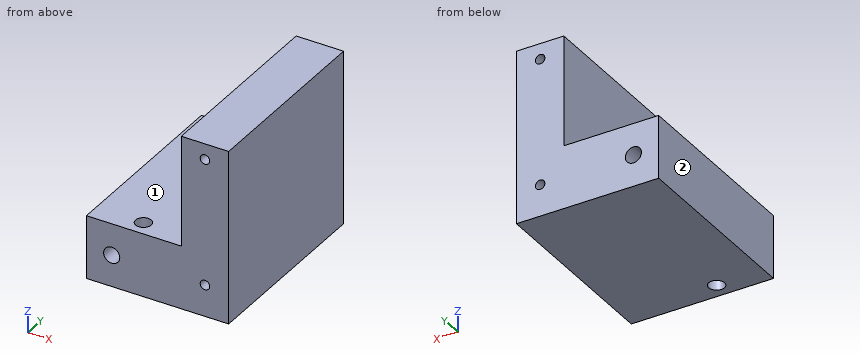
from build123d import *

# Parameters (mm, degrees)
SKETCH1_W           = 15
SKETCH1_H           = 55
SKETCH1_R           = 1.5
SKETCH1_W_2         = 30
SKETCH1_H_2         = 20
SKETCH1_R_2         = 2.55
BOSS_EXTRUDE1_DEPTH = 60
SKETCH2_R           = 2.5
CUT_EXTRUDE1_DEPTH  = 20


with BuildPart() as part:
    # Sketch1 → Boss-Extrude1 (new body)
    # profile 1 of 2: a face of its own
    with BuildSketch(Plane(origin=(0, 0, 0), x_dir=(1, 0, 0), z_dir=(0, 1, 0))):
        Rectangle(SKETCH1_W, SKETCH1_H)
        with Locations(Location((0, -22.5, 0), (0, 0, 270))):
            Circle(SKETCH1_R, mode=Mode.SUBTRACT)
        with Locations(Location((0, 17.5, 0), (0, 0, 270))):
            Circle(SKETCH1_R, mode=Mode.SUBTRACT)
    # profile 2 of 2: a face of its own
    with BuildSketch(Plane(origin=(0, 0, 0), x_dir=(1, 0, 0), z_dir=(0, 1, 0))):
        with Locations((-22.5, 17.5)):
            Rectangle(SKETCH1_W_2, SKETCH1_H_2)
        with Locations(Location((-29.5, 17.5, 0), (0, 0, 270))):
            Circle(SKETCH1_R_2, mode=Mode.SUBTRACT)
    extrude(amount=BOSS_EXTRUDE1_DEPTH)

    # Sketch2 → Cut-Extrude1 (cut)
    with BuildSketch(Plane(origin=(0, 0, -27.5), x_dir=(-1, 0, 0), z_dir=(0, 0, -1))):
        with Locations((22.5, 5)):
            Circle(SKETCH2_R)
    extrude(amount=-CUT_EXTRUDE1_DEPTH, mode=Mode.SUBTRACT)


solid = part.part
Geometry check sheet. Reference: the model listing, model coordinates, mm. Face numbers are marked on the shaded views. A direction names the side the tool comes from. Give positions to 0.01 mm unless a question says otherwise; leave off trailing zeros. Order: outer loops, then holes, each group sorted by start corner. A loop starts at its lowest first (then second) coordinate and runs counter-clockwise, first axis right, second up.
1. Sectioned sample at A-A (y = 5). Record the boundary of the cut face in (x, z).
Completed:
outline: (-37.5, -27.5) - (-25, -27.5) - (-25, -7.5) - (-37.5, -7.5) - close; (-20, -27.5) - (7.5, -27.5) - (7.5, 27.5) - (-7.5, 27.5) - (-7.5, -7.5) - (-20, -7.5) - close; hole circle Ø5.1 at (-29.5, -17.5); hole circle Ø3 at (0, -17.5); hole circle Ø3 at (0, 22.5)
2. Depth check by flat-ended pin: pin 1 (1.8 mm diameter, centred on x = 0, z = -17.5, fed in from -Y); pin 2 (4 mm diameter, centred on x = -30, z = -21, fed in from -Y); pin 3 (4 mm diameter, centred on y = 31.5, z = 13.5, fed in from -X); pin 4 (8 mm diameter, centred on x = -14.5, y = 52, fed in from +Z). Enter the tip coordinate at first touch or a pass-through.
Completed:
pin 1: passes through
pin 2: stops at y = 0
pin 3: stops at x = -7.5
pin 4: stops at z = -7.5
3. Scan lines: line 1 (X direction, y = 23.5, z = -17.5); line 2 (X direction, y = 40, z = 22.5); line 3 (X direction, y = 54.5, z = 13.5). Record each from-to range of solid material in increasing order.
Completed:
line 1: x = -37.5 to -32.05, -26.95 to -1.5, 1.5 to 7.5
line 2: x = -7.5 to -1.5, 1.5 to 7.5
line 3: x = -7.5 to 7.5
4. Sectioned sample at B-B (z = -17.5). Record the boundary of the cut face in (x, y).
Completed:
outline: (-37.5, 0) - (-32.05, 0) - (-32.05, 60) - (-37.5, 60) - close; (-26.95, 0) - (-1.5, 0) - (-1.5, 60) - (-26.95, 60) - close; (1.5, 0) - (7.5, 0) - (7.5, 60) - (1.5, 60) - close; hole circle Ø5 at (-22.5, 5)
5. Access from +Z, -Z, +X, -X, +Y, -Y to the whole of each face (thin tool, end or side, straight path). Record for the marked faces 1 and 2.
Completed:
face 1: +Z, -X, +Y, -Y
face 2: +Z, -Z, -X, +Y, -Y
6. Sectioned sample at D-D (x = 0). Record the boundary of the cut face in (y, z), then the cut area to 3 significant figures.
Completed:
outline: (0, -27.5) - (60, -27.5) - (60, -19) - (0, -19) - close; (0, -16) - (60, -16) - (60, 21) - (0, 21) - close; (0, 24) - (60, 24) - (60, 27.5) - (0, 27.5) - close
area: 2,940 mm2
7. Sectioned sample at C-C (x = -29.5). Record the boundary of the cut face in (y, z).
Completed:
outline: (0, -27.5) - (60, -27.5) - (60, -20.05) - (0, -20.05) - close; (0, -14.95) - (60, -14.95) - (60, -7.5) - (0, -7.5) - close
